For this review, take the finished solid that the model builds, in its own axes (mm). Face numbers are marked on the shaded views. A direction names the side the tool comes from. Coordinates: 2 decimals unless noted, no trailing zeros. Write each loop counter-clockwise with the first axis right and the second up, starting at its lowest first coordinate (ties: lowest second). Pieces come first, ordered by that corner, then holes.
Autodesk Inventor part; units mm, degrees
ref_plane "YZ Plane" through (0, 0, 0) normal (1, 0, 0) x (0, 1, 0)
ref_plane "XZ Plane" through (0, 0, 0) normal (0, 1, 0) x (-1, 0, 0)
ref_plane "XY Plane" through (0, 0, 0) normal (0, 0, 1) x (1, 0, 0)
sketch "Sketch1" plane through (0, 0, 0) normal (0, 0, 1) x (1, 0, 0)
  circle A0 centre (0, 0) radius 15.875
  circle A1 centre (0, 0) radius 6.35
  dimension "d0" = 31.75
  dimension "d1" = 12.7
extrude "Extrusion1" add sketch "Sketch1" along normal mid plane 50.8
sketch "Sketch2" plane through (0, 0, 25.4) normal (0, 0, 1) x (1, 0, 0)
  circle A0 centre (0, 0) radius 6.35
  circle A1 centre (0, 0) radius 25.4
  dimension "d4" = 50.8
  dimension "d7" = 12.7
extrude "Extrusion2" add sketch "Sketch2" along normal blind 6.35
mirror "Mirror1" about plane through (0, 0, 0) normal (0, 0, 1) of "Extrusion2"
properties part number "lift Hub"
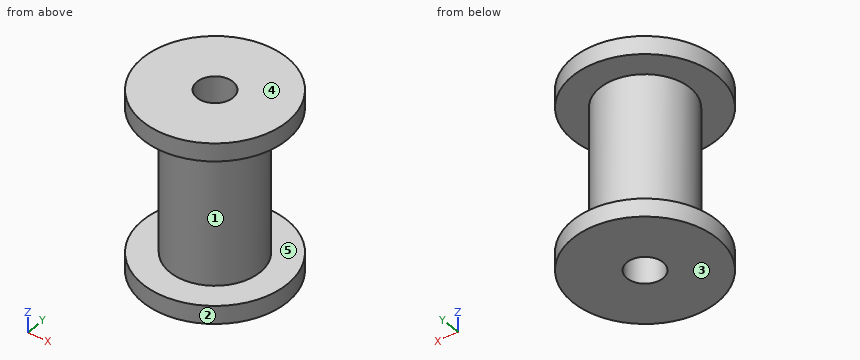
Q1. Add section C-C (z = 18). State the section outline as (x, y) points (3 decimals), then the cut area to 3 significant figures.
Ans:
outline: circle Ø31.75 at (0, 0); hole circle Ø12.7 at (0, 0)
area: 665 mm2
Q2. For probe 1 along Y at (x, z) = (0, -4.5) (3 decimals); probe 2 along Z at (x, y) = (-7.5, -16); probe 3 along X at (y, z) = (3.5, -2), list the stretches that pass through material, from the lowest coordinate up.
Ans:
probe 1: y = -15.875 to -6.35, 6.35 to 15.875
probe 2: z = -31.75 to -25.4, 25.4 to 31.75
probe 3: x = -15.48 to -5.3, 5.3 to 15.48
Q3. Draft analysis for pull direction Z (two halves, no side actions). For the marked faces 1, 2 and 3, state which applies: +Z half, -Z half, draft (parallel to the pull), parting line (faces both ways), or undercut.
Ans:
face 1: undercut
face 2: draft
face 3: -Z half
Q4. Clearance check with flat-ended pins moving along their axes: pin 1 Ø3 at (x, z) = (-2, -17) entering from +Y; pin 2 Ø10 at (y, z) = (-8, 15) entering from +X; pin 3 Ø4 at (x, z) = (12.5, -21.5) entering from -Y. State where each tip first meets the part, or that it passes through.
Ans:
pin 1: stops at y = 15.87
pin 2: stops at x = 15.59
pin 3: stops at y = -11.91
Q5. Add section A-A (x = 0). State the section outline as (y, z) points (3 decimals).
Ans:
outline: (-25.4, -31.75) - (-6.35, -31.75) - (-6.35, 31.75) - (-25.4, 31.75) - (-25.4, 25.4) - (-15.875, 25.4) - (-15.875, -25.4) - (-25.4, -25.4) - close; (6.35, -31.75) - (25.4, -31.75) - (25.4, -25.4) - (15.875, -25.4) - (15.875, 25.4) - (25.4, 25.4) - (25.4, 31.75) - (6.35, 31.75) - close
Q6. Add section D-D (x = -22). State the section outline as (y, z) points, then the cut area to 3 significant figures.
Ans:
outline: (-12.69, -31.75) - (12.69, -31.75) - (12.69, -25.4) - (-12.69, -25.4) - close; (-12.69, 25.4) - (12.69, 25.4) - (12.69, 31.75) - (-12.69, 31.75) - close
area: 322 mm2
Q7. Tool access review of the marked faces 4 and 5: name each direction out of +Z, -Z, +X, -X, +Y, -Y from which nothing blocks a thin tool from reaching the whole face with its end or side.
Ans:
face 4: +Z, +X, -X, +Y, -Y
face 5: none
